Source: CAD feature listing. Evaluate the final solid. Frame: model axes, mm. Face numbers are marked on the shaded views. A direction names the side the tool comes from. Coordinates: 2 decimals unless noted, no trailing zeros. Order: outer loops, then holes, each group sorted by start corner. A loop starts at its lowest first (then second) coordinate and runs counter-clockwise, first axis right, second up. Notation, with made-up numbers: (-5.5, -11) -> (20.5, -11) arc R22 ccw to (20.5, 24) -> close; hole circle Ø1 at (-28, 50). An arc over 180 degrees is marked (long way). Put each result on its own line as item: value.
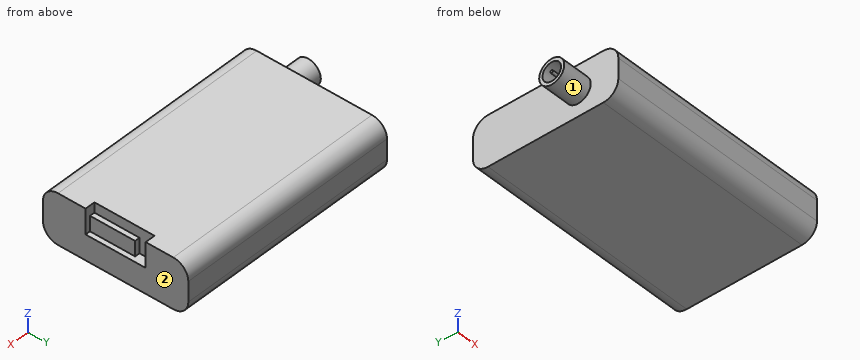
from build123d import *

# Parameters (mm, degrees)
SKETCH1_W           = 45
SKETCH1_H           = 29
BOSS_EXTRUDE1_DEPTH = 10
SKETCH2_W           = 2
SKETCH2_H           = 12
CUT_EXTRUDE1_DEPTH  = 5
SKETCH3_W           = 3
SKETCH3_H           = 9
BOSS_EXTRUDE2_DEPTH = 1
SKETCH4_R           = 2.5
BOSS_EXTRUDE3_DEPTH = 6
SKETCH5_R           = 1.85
CUT_EXTRUDE2_DEPTH  = 4
SKETCH6_R           = 0.275
BOSS_EXTRUDE4_DEPTH = 4
FILLET2_R           = 3
FILLET3_R           = 3
FILLET4_R           = 3
FILLET5_R           = 3


with BuildPart() as part:
    # Sketch1 → Boss-Extrude1 (new body)
    with BuildSketch(Plane.XY):
        Rectangle(SKETCH1_W, SKETCH1_H)
    extrude(amount=BOSS_EXTRUDE1_DEPTH)

    # Sketch2 → Cut-Extrude1 (cut)
    with BuildSketch(Plane.XY.offset(10)):
        with Locations((21.5, 0)):
            Rectangle(SKETCH2_W, SKETCH2_H)
    extrude(amount=-CUT_EXTRUDE1_DEPTH, mode=Mode.SUBTRACT)

    # Sketch3 → Boss-Extrude2 (add)
    with BuildSketch(Plane(origin=(20.5, 0, 0), x_dir=(0, 0, -1), z_dir=(1, 0, 0))):
        with Locations((-6.5, -1.5)):
            Rectangle(SKETCH3_W, SKETCH3_H)
    extrude(amount=BOSS_EXTRUDE2_DEPTH)

    # Sketch4 → Boss-Extrude3 (add)
    with BuildSketch(Plane.ZY.offset(22.5)):
        with Locations(Location((5, -6.5, 0), (0, 0, 180))):
            Circle(SKETCH4_R)
    extrude(amount=BOSS_EXTRUDE3_DEPTH)

    # Sketch5 → Cut-Extrude2 (cut)
    with BuildSketch(Plane.ZY.offset(28.5)):
        with Locations((5, -6.5)):
            Circle(SKETCH5_R)
    extrude(amount=-CUT_EXTRUDE2_DEPTH, mode=Mode.SUBTRACT)

    # Sketch6 → Boss-Extrude4 (add)
    with BuildSketch(Plane.ZY.offset(24.5)):
        with Locations((5, -6.5)):
            Circle(SKETCH6_R)
    extrude(amount=BOSS_EXTRUDE4_DEPTH)

    # Fillet2
    fillet2_edges = [part.edges().sort_by_distance(p)[0] for p in [
        (0, 14.5, 0),
    ]]
    fillet(fillet2_edges, radius=FILLET2_R)

    # Fillet3
    fillet3_edges = [part.edges().sort_by_distance(p)[0] for p in [
        (0, 14.5, 10),
    ]]
    fillet(fillet3_edges, radius=FILLET3_R)

    # Fillet4
    fillet4_edges = [part.edges().sort_by_distance(p)[0] for p in [
        (0, -14.5, 0),
    ]]
    fillet(fillet4_edges, radius=FILLET4_R)

    # Fillet5
    fillet5_edges = [part.edges().sort_by_distance(p)[0] for p in [
        (0, -14.5, 10),
    ]]
    fillet(fillet5_edges, radius=FILLET5_R)


solid = part.part
1. Cut plane D-D on y = 11. Output: boundary loops of the cut face in (x, z).
Numbers:
outline: (-22.5, 0) -> (22.5, 0) -> (22.5, 10) -> (-22.5, 10) -> close
2. First-contact query: pin 1 (1.5 mm diameter, centred on y = -1.5, z = 6, fed in from +X); pin 2 (1 mm diameter, centred on x = 22, z = 8.5, fed in from -Y); pin 3 (0.6 mm diameter, centred on x = 21.5, y = -2.5, fed in from +Z). Flat tips, straight axial feed; report the tip coordinate or a pass-through.
Numbers:
pin 1: stops at x = 21.5
pin 2: stops at y = -14.33
pin 3: stops at z = 8
3. Ray query, line 1 along Y through (x, z) = (-26.7, 5) (3 decimals); line 2 along X through (y, z) = (-9.5, 3.5); line 3 along X through (y, z) = (-2.25, 9). Return the intervals inside material, ascending.
Numbers:
line 1: y = -9 to -8.35, -6.775 to -6.225, -4.65 to -4
line 2: x = -22.5 to 22.5
line 3: x = -22.5 to 20.5
4. Cut plane B-B on x = -9.5. Output: boundary loops of the cut face in (y, z), plus the area to 3 significant figures.
Numbers:
outline: (-14.5, 3) arc R3 ccw to (-11.5, 0) -> (11.5, 0) arc R3 ccw to (14.5, 3) -> (14.5, 7) arc R3 ccw to (11.5, 10) -> (-11.5, 10) arc R3 ccw to (-14.5, 7) -> close
area: 282 mm2
5. Cut plane A-A on y = 0. Output: boundary loops of the cut face in (x, z).
Numbers:
outline: (-22.5, 0) -> (22.5, 0) -> (22.5, 5) -> (21.5, 5) -> (21.5, 8) -> (20.5, 8) -> (20.5, 10) -> (-22.5, 10) -> close
6. Set-up query: the marked faces 1 and 2. Return all of +Z, -Z, +X, -X, +Y, -Y with unobstructed straight access to the full face (end or side cutting, diameter ignored); none if empty.
Numbers:
face 1: -X
face 2: +Z, -Z, +X, +Y, -Y
7. Cut plane C-C on y = 4.5. Output: boundary loops of the cut face in (x, z), plus the area to 3 significant figures.
Numbers:
outline: (-22.5, 0) -> (22.5, 0) -> (22.5, 5) -> (20.5, 5) -> (20.5, 10) -> (-22.5, 10) -> close
area: 440 mm2
